Source: CAD feature listing. Evaluate the final solid. Frame: model axes, mm. A direction names the side the tool comes from. Round coordinates to 2 decimals unless told otherwise and drop trailing zeros. Loops run counter-clockwise (first coordinate to the right, second up) from the corner with the lowest first, then second, coordinate; pieces in that order, holes last. Notation, with made-up numbers: (-10, -25) - (-2, -25) arc R27 ccw to (-2, 2) - close; hole circle Ø3 at (41, -20). An arc over 180 degrees is marked (long way). One line per question, with ' | ' between items. Start each with the question number.
1. Ray query, line 1 (Y direction, x = 55, z = 10.5); line 2 (Y direction, x = 20.5, z = 0.45); line 3 (Z direction, x = 20, y = -95.5). Return the intervals inside material, ascending.
2. Access query for faces 1 (the flat face through (54, -83, 1)), 2 (the cylindrical face through (90.423, -32.274, 0.493)). Directions: +Z, -Z, +X, -X, +Y, -Y. A direction counts if a zero-diameter tool reaches every point of the face in a straight line with its end or side. Return the directions, or none.
3. Cut plane A-A (x = 89.5). Return loops of the section in (y, z), then the cut area to 3 significant figures.
4. Cut plane C-C (y = -55). Return loops of the section in (x, z).
5. Mould query, pull axis X, two halves, no side actions, for faces 3 (the cylindrical face through (20.066, -32.452, 0.493)), 4 (the flat face through (54, -1, 7)), 5 (the flat face through (110, -84.4, 0.6)), 6 (the cylindrical face through (21.423, -139.274, 0.493)). Classes: pulls with the +X half, pulls with the -X half, needs draft (parallel to the pull), parting line crosses it, or undercut.
6. Pin query (flat end, axial travel): pin 1 (2.5 mm diameter, centred on x = 5, z = 6.6, fed in from -Y); pin 2 (5 mm diameter, centred on x = 89.5, y = -137.5, fed in from +Z). Return the tip coordinate at first contact, or that it passes through.
7. Cut plane B-B (y = -30.5). Return loops of the section in (x, z).
```python
from build123d import *

# Parameters (mm, degrees)
ESQUISSE1_W             = 110
ESQUISSE1_H             = 168
ESQUISSE1_R             = 2
BOSS_EXTRU_1_DEPTH      = 1
ESQUISSE2_W             = 110
ESQUISSE2_H             = 1
BOSS_EXTRU_2_DEPTH      = 10.6
CONG_1_R                = 2
CONG_2_R                = 1
ESQUISSE3_R             = 1.5
ENL_V_MAT_EXTRU_1_DEPTH = 202.143133117


with BuildPart() as part:
    # Esquisse1 → Boss.-Extru.1 (new body)
    with BuildSketch(Plane.XY):
        with Locations((55, -84)):
            Rectangle(ESQUISSE1_W, ESQUISSE1_H)
        with Locations((20.5, -30.5)):
            Circle(ESQUISSE1_R, mode=Mode.SUBTRACT)
        with Locations((89.5, -30.5)):
            Circle(ESQUISSE1_R, mode=Mode.SUBTRACT)
        with Locations((89.5, -137.5)):
            Circle(ESQUISSE1_R, mode=Mode.SUBTRACT)
        with Locations((20.5, -137.5)):
            Circle(ESQUISSE1_R, mode=Mode.SUBTRACT)
    extrude(amount=BOSS_EXTRU_1_DEPTH)

    # Esquisse2 → Boss.-Extru.2 (add)
    with BuildSketch(Plane.XY.offset(1)):
        with Locations((55, -167.5)):
            Rectangle(ESQUISSE2_W, ESQUISSE2_H)
        with Locations((55, -0.5)):
            Rectangle(ESQUISSE2_W, ESQUISSE2_H)
    extrude(amount=BOSS_EXTRU_2_DEPTH)

    # Congé1
    cong_1_edges = [part.edges().sort_by_distance(p)[0] for p in [
        (55, 0, 0),
        (55, -168, 0),
    ]]
    fillet(cong_1_edges, radius=CONG_1_R)

    # Congé2
    cong_2_edges = [part.edges().sort_by_distance(p)[0] for p in [
        (55, -167, 1),
        (55, -1, 1),
    ]]
    fillet(cong_2_edges, radius=CONG_2_R)

    # Esquisse3 → Enlèv. mat.-Extru.1 (cut, through all)
    with BuildSketch(Plane(origin=(0, 0, 0), x_dir=(1, 0, 0), z_dir=(0, 1, 0))):
        with Locations(Location((105, -6.6, 0), (0, 0, 270))):
            Circle(ESQUISSE3_R)
        with Locations(Location((5, -6.6, 0), (0, 0, 270))):
            Circle(ESQUISSE3_R)
    extrude(amount=-ENL_V_MAT_EXTRU_1_DEPTH, mode=Mode.SUBTRACT)


solid = part.part
```
Answers follow:
1) line 1: y = -168 to -167, -1 to 0 | line 2: y = -167.26 to -139.5, -135.5 to -32.5, -28.5 to -0.74 | line 3: z = 0 to 1
2) face 1: +Z, +X, -X | face 2: +Z, -Z
3) outline: (-168, 2) arc R2 ccw to (-166, 0) - (-139.5, 0) - (-139.5, 1) - (-166, 1) arc R1 cw to (-167, 2) - (-167, 11.6) - (-168, 11.6) - close; (-135.5, 0) - (-32.5, 0) - (-32.5, 1) - (-135.5, 1) - close; (-28.5, 0) - (-2, 0) arc R2 ccw to (0, 2) - (0, 11.6) - (-1, 11.6) - (-1, 2) arc R1 cw to (-2, 1) - (-28.5, 1) - close | area: 180 mm2
4) outline: (0, 0) - (110, 0) - (110, 1) - (0, 1) - close
5) face 3: undercut | face 4: needs draft | face 5: pulls with the +X half | face 6: undercut
6) pin 1: passes through | pin 2: stops at z = 1
7) outline: (0, 0) - (18.5, 0) - (18.5, 1) - (0, 1) - close; (22.5, 0) - (87.5, 0) - (87.5, 1) - (22.5, 1) - close; (91.5, 0) - (110, 0) - (110, 1) - (91.5, 1) - close
